Read the model definition and answer for the solid it produces. Units are mm, in the model's axes. Coordinates: 2 decimals unless noted, no trailing zeros. Write each loop counter-clockwise with the first axis right and the second up, starting at its lowest first coordinate (ties: lowest second). Pieces come first, ordered by that corner, then holes. Notation, with made-up numbers: (44, 15.5) -> (88, 15.5) arc R23 ccw to (88, 44.5) -> close; hole circle Ø4 at (-33.75, 35). An arc over 180 degrees is marked (long way). Answer in a Markdown table with one row per item. Add a question column.
Item 1: Section C-C on y = 5.5 is taken. Count the separate pieces of the cut face and the enclosed holes in it, then the cut area to 3 significant figures.
Item 2: Straight lines are drawn through the part: line 1 (Z direction, x = -118, y = 8.5); line 2 (Z direction, x = 70, y = 13.5); line 3 (X direction, y = -3.5, z = 10). For each, find the intervals that lie inside material, in ascending order. Write a range as from..to.
Item 3: Section B-B on x = -80 is taken. Write down the section's boundary in (y, z) (3 decimals), then the cut area to 3 significant figures.
Item 4: For a pull along X with two mould halves and no side action, classify faces 1 (the face through (137.052, 0.291, -26.461)), 2 (the face through (-153.26, -20.72, -25.28)), 3 (the face through (112.77, 0.29, 17.89)), 4 (the face through (161.6, 17.9, 0.3)) as +X half, -X half, draft (parallel to the pull), parting line (faces both ways), or undercut.
Item 5: Given pin 1 Ø6 at (x, y) = (131, 11) entering from +Z; pin 2 Ø2 at (x, z) = (70.5, 16.45) entering from -Y; pin 3 Ø10 at (y, z) = (10.5, -27.5) entering from -X; pin 4 Ø6 at (x, z) = (152.03, -18.03) entering from -Y, each flat-ended and moving along its own axis, determine where each tip first touches the part or whether it passes through.
Item 6: Section A-A on z = -47.5 is taken. Write down the section's boundary in (x, y).
```python
from build123d import *

# Parameters (mm, degrees)
SKETCH1_R                      = 20.1
SKETCH1_R_2                    = 15.875
BOSS_EXTRUDE1_DEPTH            = 21
CUT_EXTRUDE3_DEPTH             = 182.833027803
MIRROR2_COPY_1_DEPTH           = 182.833027803
M6_CLEARANCE_HOLE1_D           = 6.4
CHAMFER2_SIZE                  = 0.5
CHAMFER5_SIZE                  = 1
CHAMFER6_SIZE                  = 0.5
M3X0_5_TAPPED_HOLE1_AT_2_COUNT = 2
M3X0_5_TAPPED_HOLE1_AT_2_PITCH = 32.908965344
M3X0_5_TAPPED_HOLE1_AT_3_COUNT = 2
M3X0_5_TAPPED_HOLE1_AT_3_PITCH = 32.908965344
CHAMFER9_SIZE                  = 0.2


with BuildPart() as part:
    # Sketch1 → Boss-Extrude1 (new, symmetric)
    with BuildSketch(Plane(origin=(0, 0, 0), x_dir=(1, 0, 0), z_dir=(0, 1, 0))):
        with BuildLine():
            Line((-146.444734798, 30.022967472), (-53.677446084, 68.47567229))
            ThreePointArc((-53.677446084, 68.47567229), (-49.92341171, 69.615216616), (-46.019147746, 70))
            Line((-46.019147746, 70), (46.019147746, 70))
            ThreePointArc((46.019147746, 70), (49.92341171, 69.615216616), (53.677446084, 68.47567229))
            Line((53.677446084, 68.47567229), (146.444734798, 30.022967472))
            ThreePointArc((146.444734798, 30.022967472), (166.5, 0), (146.444734798, -30.022967472))
            Line((146.444734798, -30.022967472), (53.677446084, -68.47567229))
            ThreePointArc((53.677446084, -68.47567229), (49.92341171, -69.615216616), (46.019147746, -70))
            Line((46.019147746, -70), (-46.019147746, -70))
            ThreePointArc((-46.019147746, -70), (-49.92341171, -69.615216616), (-53.677446084, -68.47567229))
            Line((-53.677446084, -68.47567229), (-146.444734798, -30.022967472))
            ThreePointArc((-146.444734798, -30.022967472), (-166.5, 0), (-146.444734798, 30.022967472))
        make_face()
        with Locations(Location((-134, 0, 0), (0, 0, 90))):
            Circle(SKETCH1_R, mode=Mode.SUBTRACT)
        with Locations(Location((134, 0, 0), (0, 0, 90))):
            Circle(SKETCH1_R, mode=Mode.SUBTRACT)
        with Locations(Location((-80, 0, 0), (0, 0, 90))):
            Circle(SKETCH1_R_2, mode=Mode.SUBTRACT)
        with Locations(Location((80, 0, 0), (0, 0, 90))):
            Circle(SKETCH1_R_2, mode=Mode.SUBTRACT)
    extrude(amount=BOSS_EXTRUDE1_DEPTH, both=True)

    # Sketch5 → Cut-Extrude3 (cut, symmetric)
    with BuildSketch(Plane.XY):
        Polygon((158.5, -21), (166.5, -13), (166.5, -21), align=None)
    cut_extrude3 = extrude(amount=CUT_EXTRUDE3_DEPTH, both=True, mode=Mode.SUBTRACT)

    # Mirror1: Cut-Extrude3 across plane
    add(cut_extrude3.mirror(Plane.ZX), mode=Mode.SUBTRACT)

    # Mirror2: Cut-Extrude3 across plane
    add(cut_extrude3.mirror(Plane(origin=(0, 0, 0), x_dir=(0, 0, 1), z_dir=(1, 0, 0))), mode=Mode.SUBTRACT)

    # Mirror2 copy 1 sketch → Mirror2 copy 1 (cut, symmetric)
    with BuildSketch(Plane(origin=(0, 0, 0), x_dir=(-1, 0, 0), z_dir=(0, 0, 1))):
        Polygon((158.5, -21), (166.5, -13), (166.5, -21), align=None)
    extrude(amount=MIRROR2_COPY_1_DEPTH, both=True, mode=Mode.SUBTRACT)

    # M6 Clearance Hole1 (through all)
    with Locations(Plane(origin=(0, -21, 0), x_dir=(-1, 0, 0), z_dir=(0, -1, 0))):
        with Locations((-115.96877708, -18.03122292), (-134, -25.5), (-152.03122292, -18.03122292), (-152.03122292, 18.03122292), (-134, 25.5), (-115.96877708, 18.03122292)):
            m6_clearance_hole1 = Hole(M6_CLEARANCE_HOLE1_D / 2)

    # Mirror5: M6 Clearance Hole1 across plane
    add(m6_clearance_hole1.mirror(Plane(origin=(0, 0, 0), x_dir=(0, 0, 1), z_dir=(1, 0, 0))), mode=Mode.SUBTRACT)

    # Chamfer2
    chamfer2_edges = [part.edges().sort_by_distance(p)[0] for p in [
        (-134, -21, 20.1),
        (-134, 21, 20.1),
        (134, -21, 20.1),
        (134, 21, 20.1),
    ]]
    chamfer(chamfer2_edges, length=CHAMFER2_SIZE)

    # Chamfer5
    chamfer5_edges = [part.edges().sort_by_distance(p)[0] for p in [
        (152.974072526, -21, -26.386257252),
        (-152.974072526, -21, -26.386257252),
        (100.061090441, -21, -49.249319881),
        (-100.061090441, -21, -49.249319881),
        (49.92341171, -21, -69.615216616),
        (-49.92341171, -21, -69.615216616),
        (0, -21, -70),
        (-152.974072526, -21, 26.386257252),
        (152.974072526, -21, 26.386257252),
        (-100.061090441, -21, 49.249319881),
        (100.061090441, -21, 49.249319881),
        (-49.92341171, -21, 69.615216616),
        (49.92341171, -21, 69.615216616),
        (0, -21, 70),
        (152.974072526, 21, -26.386257252),
        (-152.974072526, 21, -26.386257252),
        (100.061090441, 21, -49.249319881),
        (-100.061090441, 21, -49.249319881),
        (49.92341171, 21, -69.615216616),
        (-49.92341171, 21, -69.615216616),
        (0, 21, -70),
        (-152.974072526, 21, 26.386257252),
        (152.974072526, 21, 26.386257252),
        (-100.061090441, 21, 49.249319881),
        (100.061090441, 21, 49.249319881),
        (-49.92341171, 21, 69.615216616),
        (49.92341171, 21, 69.615216616),
        (0, 21, 70),
    ]]
    chamfer(chamfer5_edges, length=CHAMFER5_SIZE)

    # Chamfer6
    chamfer6_edges = [part.edges().sort_by_distance(p)[0] for p in [
        (-80, -21, 15.875),
        (-80, 21, 15.875),
        (80, -21, 15.875),
        (80, 21, 15.875),
    ]]
    chamfer(chamfer6_edges, length=CHAMFER6_SIZE)

    # Sketch13 → M3x0.5 Tapped Hole1 (revolve, cut)
    with BuildSketch(Plane(origin=(99, 21, 0), x_dir=(0, 0, 1), z_dir=(1, 0, 0))):
        Polygon((0, 0), (0, 8.251075774), (1.25, 7.5), (1.25, 0), align=None)
    m3x0_5_tapped_hole1 = revolve(axis=Axis((99, 27.35, 0), (0, -1, 0)), mode=Mode.SUBTRACT)

    # M3x0.5 Tapped Hole1 at 2: M3x0.5 Tapped Hole1 ×2
    with Locations(*[Vector(-0.8660254037844387, 0, 0.5000000000000001) * (i * M3X0_5_TAPPED_HOLE1_AT_2_PITCH) for i in range(1, M3X0_5_TAPPED_HOLE1_AT_2_COUNT)]):
        add(m3x0_5_tapped_hole1, mode=Mode.SUBTRACT)

    # M3x0.5 Tapped Hole1 at 3: M3x0.5 Tapped Hole1 ×2
    with Locations(*[Vector(-0.8660254037844387, 0, -0.5000000000000001) * (i * M3X0_5_TAPPED_HOLE1_AT_3_PITCH) for i in range(1, M3X0_5_TAPPED_HOLE1_AT_3_COUNT)]):
        add(m3x0_5_tapped_hole1, mode=Mode.SUBTRACT)

    # Mirror6: M3x0.5 Tapped Hole1 across plane
    add(m3x0_5_tapped_hole1.mirror(Plane(origin=(0, 0, 0), x_dir=(0, 0, 1), z_dir=(1, 0, 0))), mode=Mode.SUBTRACT)

    # Mirror6 copy 1 sketch → Mirror6 copy 1 (revolve, cut)
    with BuildSketch(Plane(origin=(-70.5, 21, 16.454482672), x_dir=(0, 0, 1), z_dir=(-1, 0, 0))):
        Polygon((0, 0), (0, -8.251075774), (1.25, -7.5), (1.25, 0), align=None)
    revolve(axis=Axis((-70.5, 27.35, 16.454482672), (0, 1, 0)), mode=Mode.SUBTRACT)

    # Mirror6 copy 2 sketch → Mirror6 copy 2 (revolve, cut)
    with BuildSketch(Plane(origin=(-70.5, 21, -16.454482672), x_dir=(0, 0, 1), z_dir=(-1, 0, 0))):
        Polygon((0, 0), (0, -8.251075774), (1.25, -7.5), (1.25, 0), align=None)
    revolve(axis=Axis((-70.5, 27.35, -16.454482672), (0, 1, 0)), mode=Mode.SUBTRACT)

    # Mirror7: M3x0.5 Tapped Hole1 across plane
    add(m3x0_5_tapped_hole1.mirror(Plane.ZX), mode=Mode.SUBTRACT)

    # Mirror7 copy 1 sketch → Mirror7 copy 1 (revolve, cut)
    with BuildSketch(Plane(origin=(70.5, -21, 16.454482672), x_dir=(0, 0, 1), z_dir=(1, 0, 0))):
        Polygon((0, 0), (0, -8.251075774), (1.25, -7.5), (1.25, 0), align=None)
    revolve(axis=Axis((70.5, -27.35, 16.454482672), (0, -1, 0)), mode=Mode.SUBTRACT)

    # Mirror7 copy 2 sketch → Mirror7 copy 2 (revolve, cut)
    with BuildSketch(Plane(origin=(70.5, -21, -16.454482672), x_dir=(0, 0, 1), z_dir=(1, 0, 0))):
        Polygon((0, 0), (0, -8.251075774), (1.25, -7.5), (1.25, 0), align=None)
    revolve(axis=Axis((70.5, -27.35, -16.454482672), (0, -1, 0)), mode=Mode.SUBTRACT)

    # Mirror7 copy 3 sketch → Mirror7 copy 3 (revolve, cut)
    with BuildSketch(Plane(origin=(-99, -21, 0), x_dir=(0, 0, 1), z_dir=(-1, 0, 0))):
        Polygon((0, 0), (0, 8.251075774), (1.25, 7.5), (1.25, 0), align=None)
    revolve(axis=Axis((-99, -27.35, 0), (0, 1, 0)), mode=Mode.SUBTRACT)

    # Mirror7 copy 4 sketch → Mirror7 copy 4 (revolve, cut)
    with BuildSketch(Plane(origin=(-70.5, -21, 16.454482672), x_dir=(0, 0, 1), z_dir=(-1, 0, 0))):
        Polygon((0, 0), (0, 8.251075774), (1.25, 7.5), (1.25, 0), align=None)
    revolve(axis=Axis((-70.5, -27.35, 16.454482672), (0, 1, 0)), mode=Mode.SUBTRACT)

    # Mirror7 copy 5 sketch → Mirror7 copy 5 (revolve, cut)
    with BuildSketch(Plane(origin=(-70.5, -21, -16.454482672), x_dir=(0, 0, 1), z_dir=(-1, 0, 0))):
        Polygon((0, 0), (0, 8.251075774), (1.25, 7.5), (1.25, 0), align=None)
    revolve(axis=Axis((-70.5, -27.35, -16.454482672), (0, 1, 0)), mode=Mode.SUBTRACT)

    # Chamfer9
    chamfer9_edges = [part.edges().sort_by_distance(p)[0] for p in [
        (112.76877708, -21, -18.03122292),
        (112.76877708, 21, -18.03122292),
        (130.8, -21, -25.5),
        (130.8, 21, -25.5),
        (148.83122292, -21, -18.03122292),
        (148.83122292, 21, -18.03122292),
        (148.83122292, -21, 18.03122292),
        (148.83122292, 21, 18.03122292),
        (130.8, -21, 25.5),
        (130.8, 21, 25.5),
        (112.76877708, -21, 18.03122292),
        (112.76877708, 21, 18.03122292),
        (-112.76877708, -21, -18.03122292),
        (-112.76877708, 21, -18.03122292),
        (-130.8, -21, -25.5),
        (-130.8, 21, -25.5),
        (-148.83122292, -21, -18.03122292),
        (-148.83122292, 21, -18.03122292),
        (-148.83122292, -21, 18.03122292),
        (-148.83122292, 21, 18.03122292),
        (-130.8, -21, 25.5),
        (-130.8, 21, 25.5),
        (-112.76877708, -21, 18.03122292),
        (-112.76877708, 21, 18.03122292),
    ]]
    chamfer(chamfer9_edges, length=CHAMFER9_SIZE)


solid = part.part
```
Results below:
| question | item | result |
|---|---|---|
| 1 | separate pieces | 1 |
| 1 | enclosed holes | 16 |
| 1 | area | 30,500 mm2 |
| 2 | line 1 | z = -41.81..-20.5, -15.56..-12.17, 12.17..15.56, 20.5..41.81 |
| 2 | line 2 | z = -61.71..-17.6, -15.31..-12.33, 12.33..15.31, 17.6..61.71 |
| 2 | line 3 | x = -164.92..-151.44, -116.56..-92.33, -67.67..67.67, 92.33..116.56, 151.44..164.92 |
| 3 | outline | (-21, -56.482) -> (-20, -57.565) -> (20, -57.565) -> (21, -56.482) -> (21, -16.375) -> (20.5, -15.875) -> (-20.5, -15.875) -> (-21, -16.375) -> close; (-21, 16.375) -> (-20.5, 15.875) -> (20.5, 15.875) -> (21, 16.375) -> (21, 56.482) -> (20, 57.565) -> (-20, 57.565) -> (-21, 56.482) -> close |
| 3 | area | 3,500 mm2 |
| 4 | face 1 | undercut |
| 4 | face 2 | -X half |
| 4 | face 3 | undercut |
| 4 | face 4 | +X half |
| 5 | pin 1 | stops at z = 37.67 |
| 5 | pin 2 | stops at y = -13.35 |
| 5 | pin 3 | stops at x = -157.45 |
| 5 | pin 4 | passes through |
| 6 | outline | (-104.28, -20) -> (-101.67, -21) -> (101.67, -21) -> (104.28, -20) -> (104.28, 20) -> (101.67, 21) -> (-101.67, 21) -> (-104.28, 20) -> close |
